Autodesk Inventor part; units mm, degrees
ref_plane "YZ Plane" through (0, 0, 0) normal (1, 0, 0) x (0, 1, 0)
ref_plane "XZ Plane" through (0, 0, 0) normal (0, 1, 0) x (-1, 0, 0)
ref_plane "XY Plane" through (0, 0, 0) normal (0, 0, 1) x (1, 0, 0)
sketch "Sketch1" plane through (0, 0, 0) normal (0, 1, 0) x (-1, 0, 0)
  line L0 (0, 0) -> (0, -63.881)
  line L1 (0, -63.881) -> (16.891, -63.881)
  line L2 (16.891, -63.881) -> (16.891, 0)
  line L3 (16.891, 0) -> (0, 0)
  line L4 (16.891, 0) -> (24.638, 0)
  line L5 (24.638, 0) -> (24.638, -11.43)
  line L6 (24.638, -11.43) -> (16.891, -11.43)
  line L7 (16.891, -63.881) -> (24.638, -63.881)
  line L8 (24.638, -63.881) -> (24.638, -52.451)
  line L9 (24.638, -52.451) -> (16.891, -52.451)
  dimension "d0" = 63.881
  dimension "d1" = 16.891
  dimension "d2" = 7.747
  dimension "d3" = 11.43
  dimension "d4" = 7.747
  dimension "d5" = 11.43
extrude "Extrusion1" add sketch "Sketch1" along normal blind 1.651 contours L3 L2 L1 L0
extrude "Extrusion2" add sketch "Sketch1" along normal blind 6.477 contours L4 L5 L6 L2
extrude "Extrusion3" add sketch "Sketch1" along normal blind 6.477 contours L2 L9 L8 L7
hole "Hole1" at (-8.001, 1.651, -8.89) direction (0, -1, 0) diameter 5.334 end through all
hole "Hole2" at (-8.001, 1.651, -54.991) direction (0, -1, 0) diameter 5.334 end through all
hole "Hole3" at (-5.715, 1.651, -32.131) direction (0, -1, 0) diameter 5.334 end through all
hole "Hole4" at (-20.7645, 3.2385, 0) direction (0, 0, -1) diameter 5.334 end through all
properties part number "door hinge for conveyor"
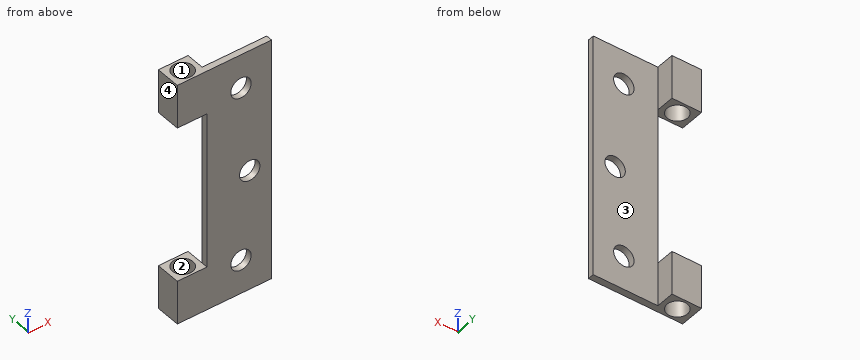
Check sheet for the modelled part. Datum: model origin and axes. Units: mm. Face numbers are marked on the shaded views. Give positions to 0.01 mm unless a question says otherwise; leave off trailing zeros. Write each loop counter-clockwise with the first axis right and the second up, starting at its lowest first coordinate (ties: lowest second). Pieces come first, ordered by that corner, then holes. Notation, with made-up numbers: (87.25, -8.75) -> (128.25, -8.75) arc R20 cw to (128.25, 1.25) -> close; hole circle Ø11 at (65, -36). An arc over 180 degrees is marked (long way). One line per item, written item: value. Start each with the question number.
Item 1: Section check A-A on z = -8.89. Record the cut outline in (x, y), then the cut area to 3 significant figures.
Item 2: Section check D-D on x = -22.25. Record the cut outline in (y, z).
Item 3: Section check B-B on y = 2.5. Record the cut outline in (x, z), then the cut area to 3 significant figures.
Item 4: Gauge pin test, flat ends, axial feed: pin 1 (0.5 mm diameter, centred on y = 0.5, z = -36, fed in from -X); pin 2 (6 mm diameter, centred on x = -19.5, z = -20, fed in from +Y); pin 3 (2.5 mm diameter, centred on y = 3, z = -7.5, fed in from +X). Record the tip position at first contact, or that the pin passes through.
Item 5: Draft check along X on the marked faces 1, 2, 3 and 4. Enter one of: +X half, -X half, draft (parallel to the pull), parting line (faces both ways), or undercut.
Item 6: Material ranges on probe 1 along X at (y, z) = (1, -11); probe 2 along X at (y, z) = (0.5, -8.89); probe 3 along Z at (x, y) = (-20.25, 6), recorded low to high. Write a range as from..to.
Item 7: Section check C-C on x = -3.75. Record the cut outline in (y, z).
Results list:
1. outline: (-24.64, 0) -> (-10.67, 0) -> (-10.67, 1.65) -> (-16.89, 1.65) -> (-16.89, 6.48) -> (-24.64, 6.48) -> close; (-5.33, 0) -> (0, 0) -> (0, 1.65) -> (-5.33, 1.65) -> close; hole circle Ø5.33 at (-20.76, 3.24)
1. area: 46.9 mm²
2. outline: (0, -63.88) -> (1.02, -63.88) -> (1.02, -52.45) -> (0, -52.45) -> close; (0, -11.43) -> (1.02, -11.43) -> (1.02, 0) -> (0, 0) -> close; (5.45, -63.88) -> (6.48, -63.88) -> (6.48, -52.45) -> (5.45, -52.45) -> close; (5.45, -11.43) -> (6.48, -11.43) -> (6.48, 0) -> (5.45, 0) -> close
3. outline: (-24.64, -63.88) -> (-23.33, -63.88) -> (-23.33, -52.45) -> (-24.64, -52.45) -> close; (-24.64, -11.43) -> (-23.33, -11.43) -> (-23.33, 0) -> (-24.64, 0) -> close; (-18.2, -63.88) -> (-16.89, -63.88) -> (-16.89, -52.45) -> (-18.2, -52.45) -> close; (-18.2, -11.43) -> (-16.89, -11.43) -> (-16.89, 0) -> (-18.2, 0) -> close
3. area: 59.9 mm²
4. pin 1: x = -16.89
4. pin 2: y = 1.65
4. pin 3: x = -16.89
5. face 1: undercut
5. face 2: undercut
5. face 3: draft
5. face 4: -X half
6. probe 1: -24.64..-22.21, -19.31..-9.63, -6.37..0
6. probe 2: -24.64..-10.67, -5.33..0
6. probe 3: -63.88..-52.45, -11.43..0
7. outline: (0, -63.88) -> (1.65, -63.88) -> (1.65, -33.93) -> (0, -33.93) -> close; (0, -30.33) -> (1.65, -30.33) -> (1.65, 0) -> (0, 0) -> close
